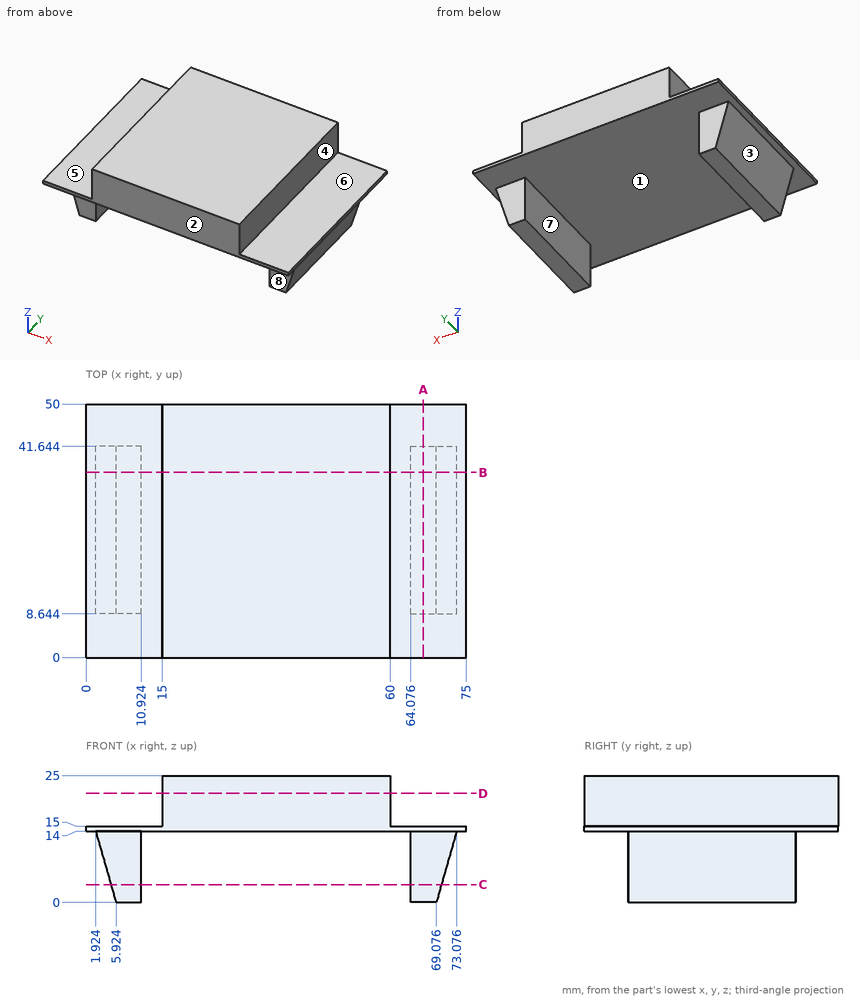
For this review, use the dimensioned drawing (mm, ordinates from the lowest corner) and the shaded views. A direction names the side the tool comes from. Coordinates: 2 decimals unless noted, no trailing zeros. Order: outer loops, then holes, each group sorted by start corner. A loop starts at its lowest first (then second) coordinate and runs counter-clockwise, first axis right, second up. Notation, with made-up numbers: M 29,44 L 83,44 A16 cw 83,51 Z; hole C 40,6 d1. An arc over 180 degrees is marked long. Answer as a JSON object with one key per item and string values. Group by question number.
1) Tool access review of the marked faces 5, 6, 7 and 8: name each direction out of +Z, -Z, +X, -X, +Y, -Y from which nothing blocks a thin tool from reaching the whole face with its end or side.
2) Add section C-C, the plane z = 3.5. Write out the cut boundary in (x, y), then the cut area to 3 significant figures.
3) Add section A-A, the plane x = 66.5. Write out the cut boundary in (y, z), then the cut area to 3 significant figures.
4) Add section D-D, the plane z = 21.5. Write out the cut boundary in (x, y).
5) Mouldability with a two-part tool opening along X and no side actions: class the marked faces 1, 2, 3 and 4 as pulls with the +X half, pulls with the -X half, needs draft (parallel to the pull), parting line crosses it, or undercut.
6) For pin 1 (25 mm diameter, centred on x = 39, y = 13, fed in from -Z); pin 2 (8 mm diameter, centred on y = 17, z = 6, fed in from -X); pin 3 (10 mm diameter, centred on x = 7.5, z = 8.5, fed in from -Y), all flat-tipped, find the tip position at first contact; note any pin that passes through.
7) Add section B-B, the plane y = 36.5. Write out the cut boundary in (x, z).
8) Wall thickness on L1, parallel to Z at x = 53, y = 42; L2, parallel to X at y = 40, z = 12 (1 decimal); L3, parallel to X at y = 43, z = 23.5: over which ranges is each line inside the solid? List them lowest first.
Computed values:
{
 "1": {"face 5": "+Z, -X, +Y, -Y", "face 6": "+Z, +X, +Y, -Y", "face 7": "-Z, +Y, -Y", "face 8": "-Z, +X, -X, -Y"},
 "2": {"outline": "M 4.92,8.64 L 10.92,8.64 L 10.92,41.64 L 4.92,41.64 Z; M 64.08,8.64 L 70.08,8.64 L 70.08,41.64 L 64.08,41.64 Z", "area": "396 mm^2"},
 "3": {"outline": "M 0,14 L 8.64,14 L 8.64,0 L 41.64,0 L 41.64,14 L 50,14 L 50,15 L 0,15 Z", "area": "512 mm^2"},
 "4": {"outline": "M 15,0 L 60,0 L 60,50 L 15,50 Z"},
 "5": {"face 1": "undercut", "face 2": "needs draft", "face 3": "pulls with the -X half", "face 4": "pulls with the +X half"},
 "6": {"pin 1": "stops at z = 14", "pin 2": "stops at x = 3.07", "pin 3": "stops at y = 8.64"},
 "7": {"outline": "M 0,14 L 1.92,14 L 5.92,0 L 10.92,0 L 10.92,14 L 64.08,14 L 64.08,0 L 69.08,0 L 73.08,14 L 75,14 L 75,15 L 60,15 L 60,25 L 15,25 L 15,15 L 0,15 Z"},
 "8": {"L1": "z = 14 to 25", "L2": "x = 2.5 to 10.9, 64.1 to 72.5", "L3": "x = 15 to 60"}
}
